```python
from build123d import *

# Parameters (mm, degrees)
SKETCH_1_W           = 85
SKETCH_1_H           = 40
EXTRUDE_1_DEPTH      = 17.5
SKETCH_2_W           = 54
SKETCH_2_H           = 20
CUT_EXTRUDE_1_DEPTH  = 4
SKETCH_3_R           = 11
CUT_EXTRUDE_2_DEPTH  = 96.557574268
SKETCH_4_W           = 41
SKETCH_4_H           = 20
CUT_EXTRUDE_3_DEPTH  = 15
CUT_EXTRUDE_4_DEPTH  = 40
SKETCH_10_R          = 2
CUT_EXTRUDE_7_DEPTH  = 3
SKETCH_8_R           = 12.5
SKETCH_8_R_2         = 11
EXTRUDE_2_DEPTH      = 7
SKETCH_12_R          = 1.25
CUT_EXTRUDE_10_DEPTH = 97.007972017


with BuildPart() as part:
    # Эскиз1 → Бобышка-Вытянуть1 (new body)
    with BuildSketch(Plane.XY):
        with Locations((42.5, -20)):
            Rectangle(SKETCH_1_W, SKETCH_1_H)
    extrude(amount=EXTRUDE_1_DEPTH)

    # Эскиз2 → Вырез-Вытянуть1 (cut)
    with BuildSketch(Plane.XY):
        with Locations((52.5, -20)):
            Rectangle(SKETCH_2_W, SKETCH_2_H)
    extrude(amount=CUT_EXTRUDE_1_DEPTH, mode=Mode.SUBTRACT)

    # Эскиз3 → Вырез-Вытянуть2 (cut, through all)
    with BuildSketch(Plane.XY):
        with Locations(Location((42.5, -20, 0), (0, 0, 245.380022671))):
            Circle(SKETCH_3_R)
    extrude(amount=CUT_EXTRUDE_2_DEPTH, mode=Mode.SUBTRACT)

    # Эскиз4 → Вырез-Вытянуть3 (cut)
    with BuildSketch(Plane.XY):
        with Locations((52, -20)):
            Rectangle(SKETCH_4_W, SKETCH_4_H)
    extrude(amount=CUT_EXTRUDE_3_DEPTH, mode=Mode.SUBTRACT)

    # Эскиз6 → Вырез-Вытянуть4 (cut)
    with BuildSketch(Plane.XZ.offset(40)):
        with BuildLine():
            Line((0, 17.5), (13.126280648, 17.5))
            ThreePointArc((13.126280648, 17.5), (6.110875281, 9.475733473), (1.230789124, 0))
            Line((1.230789124, 0), (0, 0))
            Line((0, 0), (0, 17.5))
        make_face()
        with BuildLine():
            Line((71.873719352, 17.5), (85, 17.5))
            Line((85, 17.5), (85, 0))
            Line((85, 0), (83.769210876, 0))
            ThreePointArc((83.769210876, 0), (78.889124719, 9.475733473), (71.873719352, 17.5))
        make_face()
    extrude(amount=-CUT_EXTRUDE_4_DEPTH, mode=Mode.SUBTRACT)

    # Эскиз10 → Вырез-Вытянуть7 (cut)
    with BuildSketch(Plane(origin=(0, 0, 4), x_dir=(-1, 0, 0), z_dir=(0, 0, -1))):
        with Locations((-28.5, -15)):
            Circle(SKETCH_10_R)
        with Locations((-28.5, -25)):
            Circle(SKETCH_10_R)
        with Locations((-76.5, -15)):
            Circle(SKETCH_10_R)
        with Locations((-76.5, -25)):
            Circle(SKETCH_10_R)
    extrude(amount=-CUT_EXTRUDE_7_DEPTH, mode=Mode.SUBTRACT)

    # Эскиз8 → Бобышка-Вытянуть2 (add)
    with BuildSketch(Plane.XY.offset(17.5)):
        with Locations((42.5, -20)):
            Circle(SKETCH_8_R)
        with Locations(Location((42.5, -20, 0), (0, 0, 180))):
            Circle(SKETCH_8_R_2, mode=Mode.SUBTRACT)
    extrude(amount=EXTRUDE_2_DEPTH)

    # Эскиз12 → Вырез-Вытянуть10 (cut, through all)
    with BuildSketch(Plane.XY):
        with Locations(Location((80.5, -4, 0), (0, 0, 180))):
            Circle(SKETCH_12_R)
        with Locations(Location((80.5, -36, 0), (0, 0, 180))):
            Circle(SKETCH_12_R)
        with Locations(Location((4.5, -36, 0), (0, 0, 180))):
            Circle(SKETCH_12_R)
        with Locations(Location((4.5, -4, 0), (0, 0, 180))):
            Circle(SKETCH_12_R)
    extrude(amount=CUT_EXTRUDE_10_DEPTH, mode=Mode.SUBTRACT)


solid = part.part
```
Read the model definition and answer for the solid it produces. Units are mm, in the model's axes. A direction names the side the tool comes from. Coordinates: 2 decimals unless noted, no trailing zeros. Order: outer loops, then holes, each group sorted by start corner. A loop starts at its lowest first (then second) coordinate and runs counter-clockwise, first axis right, second up. Notation, with made-up numbers: (76.25, 23) - (102.25, 23) arc R10 ccw to (102.25, 40) - close; hole circle Ø6 at (16, 38). An arc over 180 degrees is marked (long way). Answer as a JSON object with one key per item and string values. Group by question number.
Item 1: Section B-B (z = 11.25) is taken. Give the vertices of the cut face in (x, y), plus the area to 3 significant figures.
Item 2: Consider probe 1 along Y at (x, z) = (4.5, 2.25); probe 2 along Y at (x, z) = (76.5, 6); probe 3 along Y at (x, z) = (42, 10). Determine where each line is inside the solid, lowest interval first. Write a range as from..to.
Item 3: A tool of negligible diameter and unlimited length cuts with its end or side. For faces 1 (the face through (5.75, -36.05, 3.41)), 2 (the face through (32.58, -27.606, 20.951)), 3 (the face through (33, -10, 6)), from which of +Z, -Z, +X, -X, +Y, -Y can it reach the whole face along a straight path? Write none if from no direction.
Item 4: Section A-A (x = 42.5) is taken. Give the vertices of the cut face in (y, z), plus the area to 3 significant figures.
Item 5: Flat-ended cylindrical pins translate along their axes: P1, Ø5, axis at y = -35, z = 9, coming from the +X side; P2, Ø6.5, axis at x = 76.5, y = -15, coming from the +Z side; P3, Ø12, axis at x = 49, y = -18.5, coming from the -Z side; P4, Ø12, axis at x = 39.5, y = -18.5, coming from the +Z side. Find the tip coordinate at first contact, or state that the pin passes through.
Item 6: The mould has two halves that part along X. Classify faces 4 (the face through (32.207, -23.88, 17.523)), 5 (the face through (78.973, -20.28, 9.352)), 6 (the face through (24, -20, 0)): +X half, -X half, draft (parallel to the pull), parting line (faces both ways), or undercut.
Item 7: Section C-C (y = -25) is taken. Give the vertices of the cut face in (x, z), plus the area to 3 significant figures.
Item 8: Section D-D (x = 71) is taken. Give the vertices of the cut face in (y, z), plus the area to 3 significant figures.
Results are:
{
 "1": {"outline": "(7.38, -40) - (77.62, -40) - (77.62, 0) - (7.38, 0) - close; hole (31.5, -30) - (37.92, -30) arc R11 ccw to (47.08, -30) - (72.5, -30) - (72.5, -10) - (47.08, -10) arc R11 ccw to (37.92, -10) - (31.5, -10) - close", "area": "1,980 mm^2"},
 "2": {"probe 1": "y = -40..-37.25, -34.75..-5.25, -2.75..0", "probe 2": "y = -40..-27, -23..-17, -13..0", "probe 3": "y = -40..-30.99, -9.01..0"},
 "3": {"face 1": "+Z, -Z", "face 2": "+Z", "face 3": "-Z"},
 "4": {"outline": "(-40, 0) - (-31, 0) - (-31, 24.5) - (-32.5, 24.5) - (-32.5, 17.5) - (-40, 17.5) - close; (-9, 0) - (0, 0) - (0, 17.5) - (-7.5, 17.5) - (-7.5, 24.5) - (-9, 24.5) - close", "area": "336 mm^2"},
 "5": {"P1": "stops at x = 80.74", "P2": "stops at z = 16.21", "P3": "stops at z = 15", "P4": "passes through"},
 "6": {"face 4": "undercut", "face 5": "+X half", "face 6": "draft"},
 "7": {"outline": "(1.23, 0) - (25.5, 0) - (25.5, 4) - (26.5, 4) - (26.5, 7) - (30.5, 7) - (30.5, 4) - (31.5, 4) - (31.5, 15) - (32.7, 15) - (32.7, 24.5) - (31.04, 24.5) - (31.04, 17.5) - (13.13, 17.5) arc R44 ccw to start; (52.3, 15) - (72.5, 15) - (72.5, 4) - (74.5, 4) - (74.5, 7) - (78.5, 7) - (78.5, 4) - (79.5, 4) - (79.5, 0) - (83.77, 0) arc R44 ccw to (71.87, 17.5) - (53.96, 17.5) - (53.96, 24.5) - (52.3, 24.5) - close", "area": "556 mm^2"},
 "8": {"outline": "(-40, 0) - (-30, 0) - (-30, 15) - (-10, 15) - (-10, 0) - (0, 0) - (0, 17.5) - (-40, 17.5) - close", "area": "400 mm^2"}
}
